from build123d import *

# Parameters (mm, degrees)
SKETCH1_W               = 42.164
SKETCH1_H               = 42.164
BOSS_EXTRUDE1_DEPTH     = 46.7868
FILLET1_R               = 2.3622
SKETCH2_R               = 10.975
BOSS_EXTRUDE2_DEPTH     = 1.9304
SKETCH3_R               = 2.5
BOSS_EXTRUDE3_DEPTH     = 21.59
CHAMFER1_SIZE           = 0.381
SKETCH18_R              = 5.9944
SKETCH18_R_2            = 2.5
CUT_EXTRUDE8_DEPTH      = 1.524
SKETCH5_R               = 1.2446
CUT_EXTRUDE1_DEPTH      = 29.6004
CUT_EXTRUDE1_DEPTH_BACK = 42.7068
FILLET4_R               = 0.762
CHAMFER3_SIZE           = 0.508
SKETCH19_W              = 40
SKETCH19_H              = 27.280293062
CUT_EXTRUDE9_DEPTH      = 20.082


with BuildPart() as part:
    # Sketch1 → Boss-Extrude1 (new body)
    with BuildSketch(Plane(origin=(0, 0, 0), x_dir=(0, 0, -1), z_dir=(1, 0, 0))):
        Rectangle(SKETCH1_W, SKETCH1_H)
    extrude(amount=-BOSS_EXTRUDE1_DEPTH)

    # Fillet1
    fillet1_edges = [part.edges().sort_by_distance(p)[0] for p in [
        (-23.3934, 21.082, 21.082),
        (-23.3934, 21.082, -21.082),
        (-23.3934, -21.082, -21.082),
        (-23.3934, -21.082, 21.082),
    ]]
    fillet(fillet1_edges, radius=FILLET1_R)

    # Sketch2 → Boss-Extrude2 (add)
    with BuildSketch(Plane(origin=(0, 0, 0), x_dir=(0, 0, -1), z_dir=(1, 0, 0))):
        Circle(SKETCH2_R)
    extrude(amount=BOSS_EXTRUDE2_DEPTH)

    # Sketch10 → Cut-Revolve1 (revolve, cut)
    with BuildSketch(Plane.XY):
        Polygon((0, 10.975), (-0.381, 10.975), (-0.381, 11.356), (0, 11.737), align=None)
    revolve(axis=Axis((0, 0, 0), (1, 0, 0)), mode=Mode.SUBTRACT)

    # Sketch3 → Boss-Extrude3 (add)
    with BuildSketch(Plane(origin=(1.9304, 0, 0), x_dir=(0, 0, -1), z_dir=(1, 0, 0))):
        Circle(SKETCH3_R)
    extrude(amount=BOSS_EXTRUDE3_DEPTH)

    # Chamfer1
    chamfer1_edges = [part.edges().sort_by_distance(p)[0] for p in [
        (23.5204, 0, 2.5),
    ]]
    chamfer(chamfer1_edges, length=CHAMFER1_SIZE)

    # Sketch18 → Cut-Extrude8 (cut)
    with BuildSketch(Plane(origin=(1.9304, 0, 0), x_dir=(0, 0, -1), z_dir=(1, 0, 0))):
        Circle(SKETCH18_R)
        Circle(SKETCH18_R_2, mode=Mode.SUBTRACT)
    extrude(amount=-CUT_EXTRUDE8_DEPTH, mode=Mode.SUBTRACT)

    # Sketch5 → Cut-Extrude1 (cut, two sides)
    with BuildSketch(Plane(origin=(-5.08, 0, 0), x_dir=(0, 0, -1), z_dir=(1, 0, 0))) as cut_extrude1_sk:
        with Locations((-15.5, 15.5)):
            Circle(SKETCH5_R)
        with Locations((-15.5, -15.5)):
            Circle(SKETCH5_R)
        with Locations((15.5, -15.5)):
            Circle(SKETCH5_R)
        with Locations((15.5, 15.5)):
            Circle(SKETCH5_R)
    extrude(amount=CUT_EXTRUDE1_DEPTH, mode=Mode.SUBTRACT)
    extrude(cut_extrude1_sk.sketch, amount=-CUT_EXTRUDE1_DEPTH_BACK, mode=Mode.SUBTRACT)

    # Fillet4
    fillet4_edges = [part.edges().sort_by_distance(p)[0] for p in [
        (-46.7868, -21.082, 0),
        (-46.7868, 0, -21.082),
        (-46.7868, 0, 21.082),
        (-46.7868, 21.082, 0),
        (-46.7868, 20.390127639, 20.390127639),
        (-46.7868, -20.390127639, 20.390127639),
        (-46.7868, 20.390127639, -20.390127639),
        (-46.7868, -20.390127639, -20.390127639),
    ]]
    fillet(fillet4_edges, radius=FILLET4_R)

    # Chamfer3
    chamfer3_edges = [part.edges().sort_by_distance(p)[0] for p in [
        (-46.7868, 15.5, 16.7446),
        (0, 15.5, 16.7446),
        (-46.7868, -15.5, 16.7446),
        (0, -15.5, 16.7446),
        (-46.7868, -15.5, -14.2554),
        (0, -15.5, -14.2554),
        (-46.7868, 15.5, -14.2554),
        (0, 15.5, -14.2554),
    ]]
    chamfer(chamfer3_edges, length=CHAMFER3_SIZE)

    # Sketch19 → Cut-Extrude9 (cut, through all)
    with BuildSketch(Plane(origin=(0, 2, 0), x_dir=(1, 0, 0), z_dir=(0, 1, 0))):
        with Locations((23.5204, 0)):
            Rectangle(SKETCH19_W, SKETCH19_H)
    extrude(amount=CUT_EXTRUDE9_DEPTH, mode=Mode.SUBTRACT)


solid = part.part
Can you work these out from the model? Positions are in its coordinate system, mm. A direction names the side the tool comes from. Coordinates: 2 decimals unless noted, no trailing zeros. Write each loop counter-clockwise with the first axis right and the second up, starting at its lowest first coordinate (ties: lowest second). Pieces come first, ordered by that corner, then holes. Notation, with made-up numbers: (14, 2.25) -> (48, 2.25) arc R18 cw to (48, 21.25) -> close; hole circle Ø6 at (7, -2.75). An arc over 180 degrees is marked (long way). Write each question's results on one line, items separated by ' | '. Start each with the question number.
Q1. Imagine slicing it at C-C (x = 5). Write out the boundary of the cut face in (y, z).
Q2. If I drill on probe 1 along Y at (x, z) = (-2.05, 15.5); probe 2 along Y at (x, z) = (1, 0) (3 decimals); probe 3 along X at (y, z) = (-10.5, 2), over which ranges is the centre line in solid material (lowest first)?
Q3. Imagine slicing it at A-A (y = -15.5). Write out the boundary of the cut face in (x, z).
Q4. On a 3-axis mill with a long thin cutter (end or side, diameter ignored), from which of +Z, -Z, +X, -X, +Y, -Y can I reach the whole of each face in a straight line? I mean faces 4 (the face through (13, 2, 0)), 5 (the face through (-23, -21.082, 0)). Say none if no direction works.
Q5. We'd pull the mould along Y, two halves only. Please class faces 1 (the face through (0.406, 0, -3)), 2 (the face through (-23.33, 20.37, -20.41)), 3 (the face through (-23.33, -20.41, -20.37)): +Y half, -Y half, draft (parallel to the pull), parting line (faces both ways), or undercut.
Q6. I'm going to push flat-ended pins straight in: pin 1 (3 mm diameter, centred on y = 10, z = 13, fed in from +X); pin 2 (3 mm diameter, centred on y = -15.5, z = -15.5, fed in from +X); pin 3 (3 mm diameter, centred on y = -15.5, z = -15.5, fed in from -X). Where does each tip first touch, or does it pass through?
Taken from the geometry:
1) outline: (2, -1.5) -> (2, 1.5) arc R2.5 ccw (long way) to start
2) probe 1: y = -21.08 to -16.74, -14.26 to 14.26, 16.74 to 21.08 | probe 2: y = -10.975 to -5.994, -2.5 to 2.5, 5.994 to 10.975 | probe 3: x = -46.79 to 1.93
3) outline: (-46.79, -20.32) arc R0.76 ccw to (-46.02, -21.08) -> (0, -21.08) -> (0, -17.25) -> (-0.51, -16.74) -> (-46.28, -16.74) -> (-46.79, -17.25) -> close; (-46.79, -13.75) -> (-46.28, -14.26) -> (-0.51, -14.26) -> (0, -13.75) -> (0, 13.75) -> (-0.51, 14.26) -> (-46.28, 14.26) -> (-46.79, 13.75) -> close; (-46.79, 17.25) -> (-46.28, 16.74) -> (-0.51, 16.74) -> (0, 17.25) -> (0, 21.08) -> (-46.02, 21.08) arc R0.76 ccw to (-46.79, 20.32) -> close
4) face 4: +Z, -Z, +X, +Y | face 5: +Z, -Z, +X, -X, -Y
5) face 1: undercut | face 2: +Y half | face 3: -Y half
6) pin 1: stops at x = 0 | pin 2: stops at x = -0.25 | pin 3: stops at x = -46.53
